```python
from build123d import *

# Parameters (mm, degrees)
F0_R     = 19.05
F1_DEPTH = 6.35
F2_R     = 12.7
F3_DEPTH = 76.2
F4_R     = 9.398
F5_DEPTH = 7.62
F7_D     = 12.7


with BuildPart() as f1:
    # F0 (on Top) → F1 (new body)
    with BuildSketch(Plane.XY):
        Circle(F0_R)
    extrude(amount=F1_DEPTH)

    # F2 (on face) → F3 (join)
    with BuildSketch(Plane.XY.offset(6.35)):
        Circle(F2_R)
    extrude(amount=F3_DEPTH)

    # F4 (on face) → F5 (join)
    with BuildSketch(Plane.XY.offset(82.55)):
        Circle(F4_R)
    extrude(amount=F5_DEPTH)

    # F7 (through all)
    with Locations(Plane.XY.offset(90.17)):
        with Locations((0, 0)):
            Hole(F7_D / 2)


solid = f1.part
```
Geometry check sheet. Reference: the model listing, model coordinates, mm. A direction names the side the tool comes from. Coordinates: 2 decimals unless noted, no trailing zeros. Loops run counter-clockwise (first coordinate to the right, second up) from the corner with the lowest first, then second, coordinate; pieces in that order, holes last. Notation, with made-up numbers: (60, -10.75) - (72, -10.75) arc R22 ccw to (72, -2.75) - close; hole circle Ø9 at (-39.5, 66.25). An arc over 180 degrees is marked (long way). One line per item, written item: value. Start each with the question number.
(1) Mould release check, pull along X, two halves, no side actions. Record for faces 1 (the flat face through (1.8, 9.5, 82.55)), 2 (the cylindrical face through (-2.75, -12.4, 43.92)), 3 (the cylindrical face through (1.38, -6.2, 44.45)): released by +X, released by -X, zero draft, split by the parting line, or undercut.
(2) Cross-section at C-C on z = 20. Enter the section's corners in (x, y).
(3) Cross-section at D-D on y = -15. Enter the section's corners in (x, z).
(4) Material ranges on line 1 (Y direction, x = 0, z = 60); line 2 (Y direction, x = 11, z = 27); line 3 (Z direction, x = 14, y = -12.5), recorded low to high. Write a range as [from, to].
(5) Depth check by flat-ended pin: P1, Ø6, axis at x = 2, z = 23, coming from the -Y side; P2, Ø1, axis at y = -2.5, z = 67.5, coming from the -X side; P3, Ø5, axis at y = 2.5, z = 57.5, coming from the -X side; P4, Ø1.5, axis at x = 5, y = 0.5, coming from the +Z side. Enter the tip coordinate at first touch or a pass-through.
(6) Cross-section at A-A on y = 0. Enter the section's corners in (x, z), plus the area to 3 significant figures.
(7) Tool access check on faces 4 (the cylindrical face through (-1.22, 9.32, 86.31)), 5 (the flat face through (-5, 5, 0)). Record the directions out of +Z, -Z, +X, -X, +Y, -Y that give a thin tool (end or side, any length) a straight path to the whole face; none if there is none.
Results below:
1. face 1: zero draft
1. face 2: split by the parting line
1. face 3: undercut
2. outline: circle Ø25.4 at (0, 0); hole circle Ø12.7 at (0, 0)
3. outline: (-11.74, 0) - (11.74, 0) - (11.74, 6.35) - (-11.74, 6.35) - close
4. line 1: y = [-12.7, -6.35], [6.35, 12.7]
4. line 2: y = [-6.35, 6.35]
4. line 3: z = [0, 6.35]
5. P1: stops at y = -12.7
5. P2: stops at x = -12.54
5. P3: stops at x = -12.7
5. P4: passes through
6. outline: (-19.05, 0) - (-6.35, 0) - (-6.35, 90.17) - (-9.4, 90.17) - (-9.4, 82.55) - (-12.7, 82.55) - (-12.7, 6.35) - (-19.05, 6.35) - close; (6.35, 0) - (19.05, 0) - (19.05, 6.35) - (12.7, 6.35) - (12.7, 82.55) - (9.4, 82.55) - (9.4, 90.17) - (6.35, 90.17) - close
6. area: 1,180 mm2
7. face 4: +Z
7. face 5: -Z, +X, -X, +Y, -Y
